CAD build for the part. Positions are in the model's coordinates, mm. Face numbers are marked on the shaded views. A direction names the side the tool comes from. Coordinates: 2 decimals unless noted, no trailing zeros. Loops run counter-clockwise (first coordinate to the right, second up) from the corner with the lowest first, then second, coordinate; pieces in that order, holes last. Notation, with made-up numbers: (64.5, -21.5) -> (119.5, -21.5) arc R20 cw to (119.5, 10.5) -> close; hole circle Ø4 at (73.25, -12). An arc over 180 degrees is marked (long way). Write each question's results on one line, items separated by ' | '.
```python
from build123d import *

# Parameters (mm, degrees)
F1_DEPTH = 200
F2_DEPTH = 200


with BuildPart() as f1:
    # F0 (on Front) → F1 (new body)
    with BuildSketch(Plane.XZ):
        Polygon((-200.404041155, 32.3232361522), (-200.404041155, 0), (0, 0), (0, 32.3232361522), (-174.2227269083, 32.3232361522), (-138.8900934788, 278.7407568237), (0, 278.7407568237), (0, 309.5615165938), (-138.8900934788, 309.5615165938), (-167.4122055572, 419.1463837006), (0, 419.1463837006), (0, 439.6935438375), (-195.3948229849, 439.6935438375), (-195.3948229849, 419.1463837006), (-162.8617868268, 294.1511367087), align=None)
        Polygon((0, 32.3232361522), (0, 0), (199.595958845, 0), (199.595958845, 32.3232361522), (162.8617868268, 294.1511367087), (195.3948229849, 419.1463837006), (195.3948229849, 439.6935438375), (0, 439.6935438375), (0, 419.1463837006), (167.4122055572, 419.1463837006), (138.8900934788, 309.5615165938), (0, 309.5615165938), (0, 278.7407568237), (138.8900934788, 278.7407568237), (173.4622058221, 32.3232361522), align=None)
    extrude(amount=F1_DEPTH)

    # F2 (add): a face of the model
    f2_faces = [f1.faces().sort_by_distance(p)[0] for p in [
        (-194.4598808906, 0, 16.1616180761),
    ]]
    extrude(f2_faces, amount=F2_DEPTH)


solid = f1.part
```
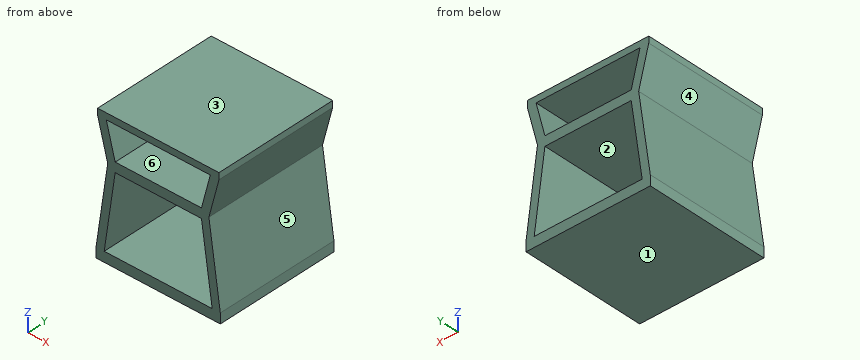
Q1. Which spindle directions (+Z, -Z, +X, -X, +Y, -Y) get a long thin tool onto all of the face, cutting with end or side? Do the marked faces 4, 5 and 6. Say none if no direction does.
Results are:
face 4: -X, +Y, -Y | face 5: +X, +Y, -Y | face 6: +Y, -Y
Q2. Cut at A-A on x = -101. Write the cut outline in (y, z).
Results are:
outline: (-200, 0) -> (200, 0) -> (200, 32.32) -> (-200, 32.32) -> close; (-200, 278.74) -> (200, 278.74) -> (200, 309.56) -> (-200, 309.56) -> close; (-200, 419.15) -> (200, 419.15) -> (200, 439.69) -> (-200, 439.69) -> close
Q3. Cut at C-C on z = 238. Write the cut outline in (x, y).
Results are:
outline: (-170.91, -200) -> (-144.73, -200) -> (-144.73, 200) -> (-170.91, 200) -> close; (144.61, -200) -> (170.74, -200) -> (170.74, 200) -> (144.61, 200) -> close
Q4. Pull direction Z, two halves, no side cores. Call the marked faces 1, 2 and 3: +Z half, -Z half, draft (parallel to the pull), parting line (faces both ways), or undercut.
Results are:
face 1: -Z half | face 2: undercut | face 3: +Z half
Q5. Cut at B-B on y = -73.5. Write the cut outline in (x, z), and give its area (3 significant figures).
Results are:
outline: (-200.4, 0) -> (199.6, 0) -> (199.6, 32.32) -> (162.86, 294.15) -> (195.39, 419.15) -> (195.39, 439.69) -> (-195.39, 439.69) -> (-195.39, 419.15) -> (-162.86, 294.15) -> (-200.4, 32.32) -> close; hole (-174.22, 32.32) -> (173.46, 32.32) -> (138.89, 278.74) -> (-138.89, 278.74) -> close; hole (-167.41, 419.15) -> (-138.89, 309.56) -> (138.89, 309.56) -> (167.41, 419.15) -> close | area: 50,100 mm^2
Q6. Drop flat-ended pins along their axis: pin 1 (10.5 mm diameter, centred on y = 32, z = 430, fed in from +X); pin 2 (12 mm diameter, centred on y = 3, z = 350, fed in from +X); pin 3 (10.5 mm diameter, centred on y = -44, z = 430.5, fed in from -X). Give the stop position or say it passes through.
Results are:
pin 1: x = 195.39 | pin 2: x = 178.96 | pin 3: x = -195.39
Q7. Wall check: L1, parallel to Z at x = 121, y = 70.5; L2, parallel to X at y = -25.5, z = 191.5; L3, parallel to X at y = -40, z = 165. Give the ranges that are in metal, low to high. Write a range as from..to.
Results are:
L1: 0..32.32, 278.74..309.56, 419.15..439.69 | L2: -177.58..-151.4, 151.13..177.26 | L3: -181.38..-155.2, 154.85..180.98
